Read the model definition and answer for the solid it produces. Units are mm, in the model's axes. Face numbers are marked on the shaded views. A direction names the side the tool comes from. Coordinates: 2 decimals unless noted, no trailing zeros. Loops run counter-clockwise (first coordinate to the right, second up) from the corner with the lowest first, then second, coordinate; pieces in that order, holes last. Notation, with made-up numbers: (47, 58) -> (62, 58) arc R6 ccw to (62, 69) -> close; hole circle Ø9 at (-38.5, -40). An arc over 180 degrees is marked (long way). Answer as a JSON object with one key per item and string values. Group by question number.
1) Section A-A, the plane x = -25 is taken. Give the vertices of the cut face in (y, z).
2) Determine the mould class of the marked faces 4, 5 and 6 for opening direction Y: released by +Y, released by -Y, zero draft, split by the parting line, or undercut.
3) Consider probe 1 along Y at (x, z) = (-23.25, 12.5); probe 2 along Y at (x, z) = (-7, 1.5); probe 3 along Z at (x, y) = (-8, 1). Determine where each line is inside the solid, lowest interval first. Write a range as [from, to].
4) Which of the six approach directions +Z, -Z, +X, -X, +Y, -Y give full straight-line access (tool end or side, diameter ignored) to the marked faces 1, 2 and 3?
5) Section D-D, the plane x = -11.5 is taken. Give the vertices of the cut face in (y, z).
6) Flat-ended cylindrical pins translate along their axes: P1, Ø2, axis at y = 5.5, z = 15.5, coming from the +X side; P2, Ø1.5, axis at y = 2.5, z = 14, coming from the -X side; P3, Ø10.5, axis at x = -3.5, z = 14.5, coming from the +Y side. Find the tip coordinate at first contact, or state that the pin passes through.
7) Section B-B, the plane y = 2 is taken. Give the vertices of the cut face in (x, z).
8) Section C-C, the plane z = 5.5 is taken. Give the vertices of the cut face in (x, y).
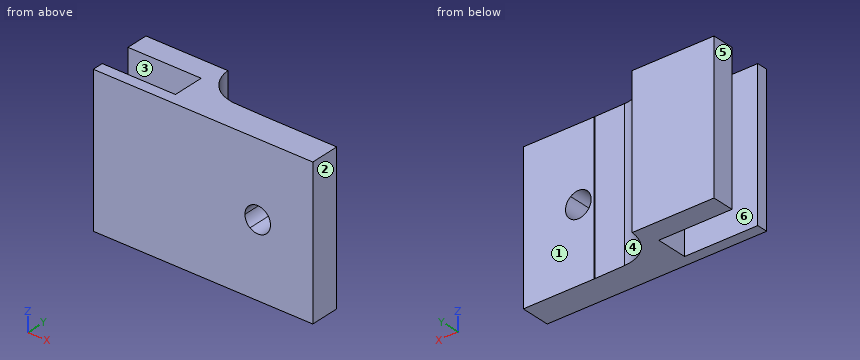
from build123d import *

# Parameters (mm, degrees)
F1_DEPTH    = 20
F2_T1_DEPTH = 20
F4_DEPTH    = 25


# Not quite as in the source:
# - a fillet or chamfer that OpenCascade refuses, or shapes differently, is made with other operations: its cross-section is extruded or revolved along the edge and cut away or added


with BuildPart() as f1:
    # F0 (on Top) → F1 (new body)
    with BuildSketch(Plane.XY):
        Polygon((-30, 0), (0, 0), (0, 1.4936865721), (0, 2.9873731442), (0, 4), (-9.7294932483, 4), (-18.8047308475, 4.1669379548), (-18.8047308475, 8.8), (-30, 8.8), (-30, 5.8), (-20, 5.8), (-20, 1.5), (-30, 1.5), align=None)
    extrude(amount=F1_DEPTH)

    # F2: fillet of radius 5 on 2 edges, made by hand

    # F2_s2 → F2_t1 (join)
    with BuildSketch(Plane.XY):
        with BuildLine():
            ThreePointArc((-9.7754687943, 4.0008457149), (-9.7294913038, 4.0002114332), (-9.6835099246, 4))
            Line((-9.6835099246, 4), (-9.7294932483, 4))
            Line((-9.7294932483, 4), (-9.7754687943, 4.0008457149))
        make_face()
        with BuildLine():
            ThreePointArc((-18.8047308475, 8.8), (-17.2821914607, 5.4759203381), (-13.904310341, 4.0767952816))
            Line((-13.904310341, 4.0767952816), (-18.8047308475, 4.1669379548))
            Line((-18.8047308475, 4.1669379548), (-18.8047308475, 8.8))
        make_face()
    extrude(amount=F2_T1_DEPTH)

    # F3 (on face) → F4 (cut)
    with BuildSketch(Plane(origin=(0, 4, 0), x_dir=(-1, 0, 0), z_dir=(0, 1, 0))):
        with BuildLine():
            Line((6.4737138013, 11.3982501667), (7.5260428712, 10))
            Line((7.5260428712, 10), (8.5783719411, 11.3982501667))
            ThreePointArc((8.5783719411, 11.3982501667), (7.5260428712, 11.75), (6.4737138013, 11.3982501667))
        make_face()
        with BuildLine():
            ThreePointArc((6.4737138013, 11.3982501667), (5.7760428712, 10), (6.4737138013, 8.6017498333))
            Line((6.4737138013, 8.6017498333), (7.5260428712, 10))
            Line((7.5260428712, 10), (6.4737138013, 11.3982501667))
        make_face()
        with BuildLine():
            Line((7.5260428712, 10), (6.4737138013, 8.6017498333))
            ThreePointArc((6.4737138013, 8.6017498333), (7.5260428712, 8.25), (8.5783719411, 8.6017498333))
            Line((8.5783719411, 8.6017498333), (7.5260428712, 10))
        make_face()
        with BuildLine():
            Line((8.5783719411, 11.3982501667), (7.5260428712, 10))
            Line((7.5260428712, 10), (8.5783719411, 8.6017498333))
            ThreePointArc((8.5783719411, 8.6017498333), (9.0919413149, 9.2186792823), (9.2760428712, 10))
            ThreePointArc((9.2760428712, 10), (9.0919413149, 10.7813207177), (8.5783719411, 11.3982501667))
        make_face()
    extrude(amount=-F4_DEPTH, mode=Mode.SUBTRACT)


solid = f1.part
Determined:
{
 "1": {"outline": "(0, 0) -> (1.5, 0) -> (1.5, 20) -> (0, 20) -> close; (5.8, 0) -> (8.8, 0) -> (8.8, 20) -> (5.8, 20) -> close"},
 "2": {"face 4": "released by +Y", "face 5": "zero draft", "face 6": "undercut"},
 "3": {"probe 1": "[0, 1.5], [5.8, 8.8]", "probe 2": "[0, 4]", "probe 3": "[0, 8.32], [11.68, 20]"},
 "4": {"face 1": "+Z, -Z, +X, +Y", "face 2": "+Z, -Z, +X, +Y, -Y", "face 3": "+Z, -Z, -X"},
 "5": {"outline": "(0, 0) -> (4.03, 0) -> (4.03, 20) -> (0, 20) -> close"},
 "6": {"P1": "x = -15.83", "P2": "x = -20", "P3": "y = 4"},
 "7": {"outline": "(-20, 0) -> (0, 0) -> (0, 20) -> (-20, 20) -> close; hole circle Ø3.5 at (-7.53, 10)"},
 "8": {"outline": "(-30, 0) -> (0, 0) -> (0, 4) -> (-9.68, 4) arc R5 cw to (-9.78, 4) -> (-13.9, 4.08) arc R5 cw to (-18.8, 8.8) -> (-30, 8.8) -> (-30, 5.8) -> (-20, 5.8) -> (-20, 1.5) -> (-30, 1.5) -> close"}
}
